Geometry check sheet. Reference: the model listing, model coordinates, mm. A direction names the side the tool comes from. Coordinates: 2 decimals unless noted, no trailing zeros. Write each loop counter-clockwise with the first axis right and the second up, starting at its lowest first coordinate (ties: lowest second). Pieces come first, ordered by that corner, then holes. Notation, with made-up numbers: M 22,38.5 L 45,38.5 A21 ccw 45,65.5 Z; hole C -18.75,45.25 d5. An arc over 180 degrees is marked long. Put each result on its own line as item: value. Start each with the question number.
1) Cross-section at B-B on z = 1. Record the cut outline in (x, y).
2) Mould release check, pull along Z, two halves, no side actions. Record for faces 1 (the flat face through (0, 6, 0)), 2 (the cylindrical face through (11.671, 4.64, 2.817)), 3 (the flat face through (2.381, 4, -2)): released by +Z, released by -Z, zero draft, split by the parting line, or undercut.
3) Gauge pin test, flat end, axial feed: pin 1 (3 mm diameter, centred on x = 13.5, y = 5, fed in from +Z). Record the tip position at first contact, or that the pin passes through.
4) Cross-section at A-A on z = 0. Record the cut outline in (x, y), plus the area to 3 significant figures.
5) Scan lines: line 1 along Z through (x, y) = (12.75, 4.5); line 2 along Z through (x, y) = (5.75, 4); line 3 along X through (y, z) = (1, -0.5). Record each from-to range of solid material in increasing order.
6) Cross-section at C-C on x = 4.5. Record the cut outline in (y, z) (3 decimals).
7) Set-up check for faces 4 (the cylindrical face through (1.174, 2.866, -2.355)), 5 (the cylindrical face through (11.64, 5.09, 0.25)), 6 (the cylindrical face through (21.811, 2.866, -2.355)): record each of +Z, -Z, +X, -X, +Y, -Y from which the full face is reachable in a straight line by a thin tool's end or side.
from build123d import *

# Parameters (mm, degrees)
F_24_0_152_DIAMETER_HOLE1_D = 3.8608


with BuildPart() as part:
    # Sketch1 → Revolve1 (revolve)
    with BuildSketch(Plane.XY, mode=Mode.PRIVATE) as revolve1_sk:
        Polygon((0, 0), (23.01875, 0), (23.01875, 0.8001), (20.6375, 0.8001), (20.6375, 3.175), (2.38125, 3.175), (2.38125, 0.8001), (0, 0.8001), align=None)
    revolve(revolve1_sk.sketch.rotate(Axis((1.613187702, 3.175, 0), (-1, 0, 0)), 180), axis=Axis((1.613187702, 3.175, 0), (-1, 0, 0)))

    # #24 (0.152) Diameter Hole1 (through all)
    with Locations(Plane.ZY.offset(-2.38125)):
        with Locations((0, 3.175)):
            Hole(F_24_0_152_DIAMETER_HOLE1_D / 2)


solid = part.part
Answer key:
1. outline: M 0,0.16 L 23.02,0.16 L 23.02,1.02 L 20.64,1.02 L 20.64,1.52 L 2.38,1.52 L 2.38,1.02 L 0,1.02 Z; M 0,5.33 L 2.38,5.33 L 2.38,4.83 L 20.64,4.83 L 20.64,5.33 L 23.02,5.33 L 23.02,6.19 L 0,6.19 Z
2. face 1: zero draft
2. face 2: split by the parting line
2. face 3: undercut
3. pin 1: stops at z = 3.16
4. outline: M 0,0 L 23.02,0 L 23.02,0.8 L 20.64,0.8 L 20.64,1.24 L 2.38,1.24 L 2.38,0.8 L 0,0.8 Z; M 0,5.55 L 2.38,5.55 L 2.38,5.11 L 20.64,5.11 L 20.64,5.55 L 23.02,5.55 L 23.02,6.35 L 0,6.35 Z
4. area: 53.1 mm²
5. line 1: z = -2.89 to -1.4, 1.4 to 2.89
5. line 2: z = -3.07 to -1.75, 1.75 to 3.07
5. line 3: x = 2.38 to 20.64
6. outline: C 3.175,0 d6.35; hole C 3.175,0 d3.861
7. face 4: -X
7. face 5: +X, -X
7. face 6: +X
